Here's the drawing with two shaded views (mm, measured from the low corner). I have some questions. A direction names the side the tool comes from. Give positions to 0.01 mm unless a question says otherwise; leave off trailing zeros. Loops run counter-clockwise (first coordinate to the right, second up) from the corner with the lowest first, then second, coordinate; pieces in that order, holes last. Notation, with made-up numbers: (13.5, 59) -> (47.5, 59) arc R34 cw to (47.5, 97) -> close; hole circle Ø8 at (-33, 75.5). An arc over 180 degrees is marked (long way). Put each result on its own line as item: value.
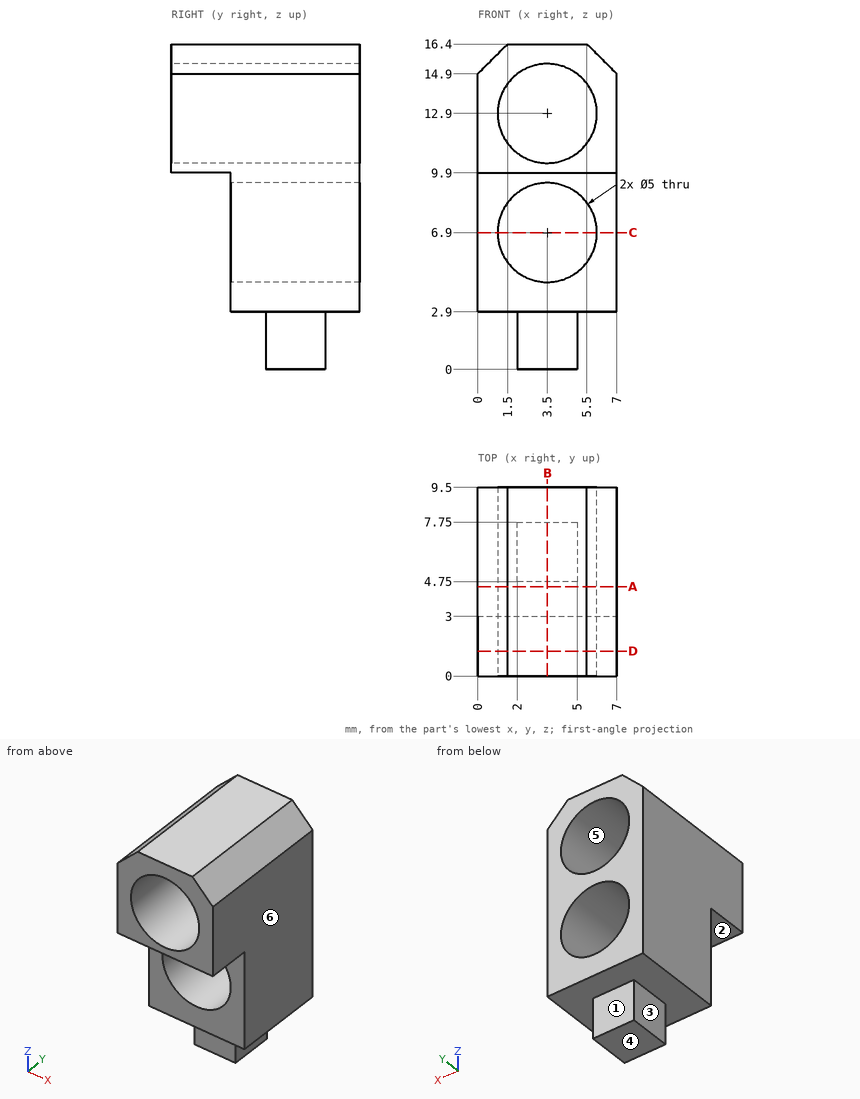
1. If we section it at D-D (y = 1.25): List the corners of the cut face in (x, z) for me.
Recorded:
outline: (0, 9.9) -> (7, 9.9) -> (7, 14.9) -> (5.5, 16.4) -> (1.5, 16.4) -> (0, 14.9) -> close; hole circle Ø5 at (3.5, 12.9)
2. I need wall thicknesses on line 1 (Z direction, x = 3.5, y = 7); line 2 (Z direction, x = 3.5, y = 2.25); line 3 (Z direction, x = 5.25, y = 6). Which ranges of each line are inside material? Lowest first, please.
Recorded:
line 1: z = 0 to 4.4, 9.4 to 10.4, 15.4 to 16.4
line 2: z = 9.9 to 10.4, 15.4 to 16.4
line 3: z = 2.9 to 5.11, 8.69 to 11.11, 14.69 to 16.4
3. If we section it at C-C (z = 6.9): List the corners of the cut face in (x, y) for me.
Recorded:
outline: (0, 3) -> (1, 3) -> (1, 9.5) -> (0, 9.5) -> close; (6, 3) -> (7, 3) -> (7, 9.5) -> (6, 9.5) -> close
4. I'm going to push flat-ended pins straight in: pin 1 (2.5 mm diameter, centred on x = 4, y = 1, fed in from -Z); pin 2 (3 mm diameter, centred on x = 4, z = 1, fed in from +Y); pin 3 (2.5 mm diameter, centred on y = 7, z = 1, fed in from -X). Where does each tip first touch, or does it pass through?
Recorded:
pin 1: stops at z = 9.9
pin 2: stops at y = 7.75
pin 3: stops at x = 2
5. For the marked faces 1, 2 and 3, which set-ups out of +Z, -Z, +X, -X, +Y, -Y let a thin tool reach every point of the face, with its end or its side?
Recorded:
face 1: -Z, +X, -X, +Y
face 2: -Z, +X, -X, -Y
face 3: -Z, -X, +Y, -Y
6. If we section it at A-A (y = 4.5): List the corners of the cut face in (x, z) for me.
Recorded:
outline: (0, 2.9) -> (7, 2.9) -> (7, 14.9) -> (5.5, 16.4) -> (1.5, 16.4) -> (0, 14.9) -> close; hole circle Ø5 at (3.5, 6.9); hole circle Ø5 at (3.5, 12.9)
7. Thinking about a two-plate mould opening in Z: for the marked faces 4, 5 and 6, which applies, pulls with the +Z half, pulls with the -Z half, needs draft (parallel to the pull), parting line crosses it, or undercut?
Recorded:
face 4: pulls with the -Z half
face 5: undercut
face 6: needs draft
8. If we section it at B-B (x = 3.5): List the corners of the cut face in (y, z) for me, then the cut area to 4 significant figures.
Recorded:
outline: (0, 9.9) -> (3, 9.9) -> (3, 9.4) -> (9.5, 9.4) -> (9.5, 10.4) -> (0, 10.4) -> close; (0, 15.4) -> (9.5, 15.4) -> (9.5, 16.4) -> (0, 16.4) -> close; (3, 2.9) -> (4.75, 2.9) -> (4.75, 0) -> (7.75, 0) -> (7.75, 2.9) -> (9.5, 2.9) -> (9.5, 4.4) -> (3, 4.4) -> close
area: 35.95 mm^2
